Check sheet for the drawn part. Datum: minimum x, y, z corner. Units: mm. A direction names the side the tool comes from. Give positions to 0.01 mm unless a question says otherwise; leave off trailing zeros. Order: outer loops, then holes, each group sorted by start corner. A loop starts at its lowest first (then second) coordinate and runs counter-clockwise, first axis right, second up. Notation, with made-up numbers: (23, 70.5) -> (55, 70.5) arc R18 cw to (55, 90.5) -> close; hole circle Ø7 at (24.5, 43). An arc over 180 degrees is marked (long way). One line per question, with ' | ' between items. Start each with the question number.
Q1. Mould release check, pull along Y, two halves, no side actions. Record for the marked faces 1, 2 and 3: released by +Y, released by -Y, zero draft, split by the parting line, or undercut.
Q2. Section check B-B on y = 5.25. Give the number of separate pieces and of enclosed holes in the cut face, plus the area to 3 significant figures.
Q3. Access from +Z, -Z, +X, -X, +Y, -Y to the whole of each face (thin tool, end or side, straight path). Record for the marked faces 4 and 5.
Q4. Section check C-C on x = 24. Record the cut outline in (y, z).
Q5. Section check A-A on x = 35. Record the cut outline in (y, z), plus the area to 3 significant figures.
Q6. Go/stop test with a flat-tipped pin: pin 1 (6.5 mm diameter, centred on x = 8.33, y = 10, fed in from -Z). Record where the tip stops, or that it passes through.
Q7. Material ranges on probe 1 along Y at (x, z) = (23, 17.5); probe 2 along Z at (x, y) = (15, 5); probe 3 along X at (y, z) = (8, 9), recorded low to high. Write a range as [from, to].
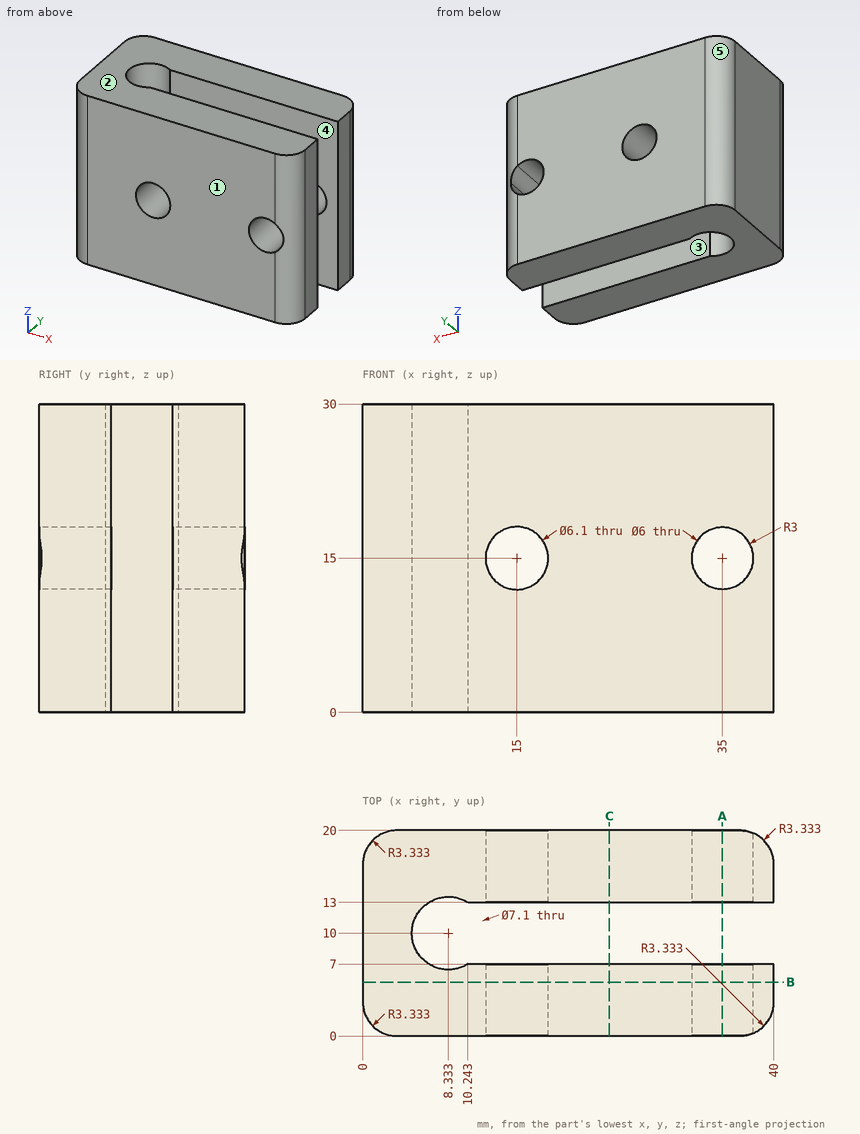
Filled in:
1) face 1: released by -Y | face 2: zero draft | face 3: undercut
2) separate pieces: 1 | enclosed holes: 2 | area: 1,140 mm²
3) face 4: +Z, -Z, +X | face 5: +Z, -Z, -X, +Y
4) outline: (0, 0) -> (7, 0) -> (7, 30) -> (0, 30) -> close; (13, 0) -> (20, 0) -> (20, 30) -> (13, 30) -> close
5) outline: (0, 0) -> (7, 0) -> (7, 12) -> (0, 12) -> close; (0, 18) -> (7, 18) -> (7, 30) -> (0, 30) -> close; (13, 0) -> (20, 0) -> (20, 12) -> (13, 12) -> close; (13, 18) -> (20, 18) -> (20, 30) -> (13, 30) -> close | area: 336 mm²
6) pin 1: through
7) probe 1: [0, 7], [13, 20] | probe 2: [0, 11.95], [18.05, 30] | probe 3: [0, 5.4]
